Work out the finished part from the listing and answer in its coordinate system (mm). A direction names the side the tool comes from. Coordinates: 2 decimals unless noted, no trailing zeros. Loops run counter-clockwise (first coordinate to the right, second up) from the corner with the lowest first, then second, coordinate; pieces in that order, holes last. Notation, with made-up numbers: (60, 0) - (119, 0) arc R22 cw to (119, 39) - close; hole circle Ø6 at (-17.5, -0.5). An arc over 180 degrees is marked (long way). Write each question's results on one line, items separated by ' | '. Start each with the question number.
1. A cutting plane is placed at A-A on y = 2. Determine the outline of the cut face in (x, z), then the cut area to 3 significant figures.
2. Find the intervals of material crossed by line 1 along X through (y, z) = (16.25, 14); line 2 along Z through (x, y) = (-13, 6.25); line 3 along X through (y, z) = (16, 14), in increasing order. Write a range as [from, to].
3. A cutting plane is placed at B-B on x = -5.5. Determine the outline of the cut face in (y, z).
4. A cutting plane is placed at C-C on x = -23.5. Determine the outline of the cut face in (y, z), then the cut area to 3 significant figures.
5. A cutting plane is placed at D-D on y = 12.75. Determine the outline of the cut face in (x, z), then the cut area to 3 significant figures.
6. Each of these flat-tipped pins is pushed along its axis until it touches: P1, Ø6.5, axis at y = 12.5, z = 6.5, coming from the +X side; P2, Ø3, axis at y = 13.5, z = 22.5, coming from the +X side; P3, Ø3, axis at x = 3.5, y = 11.5, coming from the +Z side. Where does it stop, or does it pass through?
7. Determine the mould class of faces 5 (the flat face through (0, 8, 7)), 6 (the cylindrical face through (-53.986, 8.451, 5.703)), 7 (the flat face through (-8, 9, 11)), 8 (the flat face through (-20, 8, 0)) for opening direction X: released by +X, released by -X, zero draft, split by the parting line, or undercut.
8. Which of the six approach directions +Z, -Z, +X, -X, +Y, -Y give full straight-line access (tool end or side, diameter ignored) to faces 1 (the flat face through (-11.5, 9, 13)), 2 (the flat face through (-46.054, 8.619, 14.368)), 3 (the flat face through (-56, 8, 25)), 4 (the flat face through (-25, 8, 15))?
from build123d import *

# Parameters (mm, degrees)
SALIENTE_EXTRUIR1_DEPTH  = 17
CORTAR_EXTRUIR3_DEPTH    = 40
CORTAR_REVOLUCI_N1_ANGLE = 90
CORTAR_EXTRUIR4_DEPTH    = 10
CORTAR_EXTRUIR5_DEPTH    = 27
CROQUIS15_W              = 6
CROQUIS15_H              = 17
SALIENTE_EXTRUIR2_DEPTH  = 7
CROQUIS16_W              = 2
CROQUIS16_H              = 17
SALIENTE_EXTRUIR3_DEPTH  = 7
CORTAR_EXTRUIR6_START    = -23
CROQUIS17_W              = 8
CROQUIS17_H              = 4
CORTAR_EXTRUIR6_DEPTH    = 23


with BuildPart() as part:
    # Croquis1 → Saliente-Extruir1 (new body)
    with BuildSketch(Plane(origin=(0, 0, 0), x_dir=(1, 0, 0), z_dir=(0, 1, 0))):
        with BuildLine():
            Line((0, 0), (-40, 0))
            ThreePointArc((-40, 0), (-54.142135624, -5.857864376), (-60, -20))
            Line((-60, -20), (-60, -25))
            Line((-60, -25), (0, -25))
            Line((0, -25), (0, 0))
        make_face()
    extrude(amount=SALIENTE_EXTRUIR1_DEPTH)

    # Croquis8 → Cortar-Extruir3 (cut)
    with BuildSketch(Plane(origin=(0, 0, 0), x_dir=(0, 0, -1), z_dir=(1, 0, 0))):
        with BuildLine():
            Line((-5, 0), (0, 0))
            Line((0, 0), (0, 5))
            ThreePointArc((0, 5), (-1.464466094, 1.464466094), (-5, 0))
        make_face()
        with BuildLine():
            Line((0, 12), (0, 17))
            Line((0, 17), (-5, 17))
            ThreePointArc((-5, 17), (-1.464466094, 15.535533906), (0, 12))
        make_face()
    extrude(amount=-CORTAR_EXTRUIR3_DEPTH, mode=Mode.SUBTRACT)

    # Croquis13 → Cortar-Revolución1 (revolve, cut)
    with BuildSketch(Plane(origin=(-40, 0, 0), x_dir=(0, 0, -1), z_dir=(1, 0, 0))):
        with BuildLine():
            Line((-5, 17), (0, 17))
            Line((0, 17), (0, 12))
            ThreePointArc((0, 12), (-1.464466094, 15.535533906), (-5, 17))
        make_face()
        with BuildLine():
            Line((0, 5), (0, 0))
            Line((0, 0), (-5, 0))
            ThreePointArc((-5, 0), (-1.464466094, 1.464466094), (0, 5))
        make_face()
    revolve(axis=Axis((-40, 22.120784126, 20), (0, 1, 0)), revolution_arc=CORTAR_REVOLUCI_N1_ANGLE, mode=Mode.SUBTRACT)

    # Croquis14 → Cortar-Extruir4 (cut)
    with BuildSketch(Plane(origin=(0, 0, 20), x_dir=(-1, 0, 0), z_dir=(0, 0, -1))):
        with BuildLine():
            Line((55, 17), (60, 17))
            Line((60, 17), (60, 12))
            ThreePointArc((60, 12), (58.535533906, 15.535533906), (55, 17))
        make_face()
        with BuildLine():
            Line((60, 5), (60, 0))
            Line((60, 0), (55, 0))
            ThreePointArc((55, 0), (58.535533906, 1.464466094), (60, 5))
        make_face()
    extrude(amount=-CORTAR_EXTRUIR4_DEPTH, mode=Mode.SUBTRACT)

    # Croquis12 → Cortar-Extruir5 (cut)
    with BuildSketch(Plane(origin=(0, 17, 0), x_dir=(1, 0, 0), z_dir=(0, 1, 0))):
        with BuildLine():
            Line((0, -15), (-39, -15))
            ThreePointArc((-39, -15), (-43.242640687, -16.757359313), (-45, -21))
            Line((-45, -21), (-45, -25))
            Line((-45, -25), (0, -25))
            Line((0, -25), (0, -15))
        make_face()
    extrude(amount=-CORTAR_EXTRUIR5_DEPTH, mode=Mode.SUBTRACT)

    # Croquis15 → Saliente-Extruir2 (add)
    with BuildSketch(Plane.XY.offset(25)):
        with Locations((-48, 8.5)):
            Rectangle(CROQUIS15_W, CROQUIS15_H)
    extrude(amount=SALIENTE_EXTRUIR2_DEPTH)

    # Croquis16 → Saliente-Extruir3 (add)
    with BuildSketch(Plane(origin=(0, 0, 0), x_dir=(0, 0, -1), z_dir=(1, 0, 0))):
        with Locations((-14, 8.5)):
            Rectangle(CROQUIS16_W, CROQUIS16_H)
    extrude(amount=SALIENTE_EXTRUIR3_DEPTH)

    # Croquis17 → Cortar-Extruir6 (cut)
    with BuildSketch(Plane.XZ.offset(CORTAR_EXTRUIR6_START)):
        with Locations((-7.5, 13)):
            Rectangle(CROQUIS17_W, CROQUIS17_H)
        with BuildLine():
            Line((-45, 21), (-48.843271123, 17.156728877))
            Line((-48.843271123, 17.156728877), (-43.186416873, 11.499874628))
            Line((-43.186416873, 11.499874628), (-39.650882968, 15.035408533))
            ThreePointArc((-39.650882968, 15.035408533), (-43.466838804, 16.994085486), (-45, 21))
        make_face()
    extrude(amount=CORTAR_EXTRUIR6_DEPTH, mode=Mode.SUBTRACT)


solid = part.part
Values:
1) outline: (-59, 20) arc R19 ccw to (-40, 1) - (0, 1) - (0, 13) - (7, 13) - (7, 15) - (-3.5, 15) - (-3.5, 11) - (-11.5, 11) - (-11.5, 15) - (-39, 15) arc R6 cw to (-39.65, 15.04) - (-43.19, 11.5) - (-48.84, 17.16) - (-45, 21) - (-45, 32) - (-51, 32) - (-51, 25) - (-59, 25) - close | area: 887 mm^2
2) line 1: [-56.58, -45.69], [-40.69, -11.5], [-3.5, 7] | line 2: [0, 15] | line 3: [-56.97, -45.69], [-40.69, -11.5], [-3.5, 7]
3) outline: (0, 5) arc R5 ccw to (5, 0) - (12, 0) arc R5 ccw to (17, 5) - (17, 11) - (0, 11) - close
4) outline: (0, 5) arc R5 ccw to (5, 0) - (12, 0) arc R5 ccw to (17, 5) - (17, 15) - (0, 15) - close | area: 244 mm^2
5) outline: (-59.94, 20) arc R19.94 ccw to (-40, 0.06) - (0, 0.06) - (0, 13) - (7, 13) - (7, 15) - (-3.5, 15) - (-3.5, 11) - (-11.5, 11) - (-11.5, 15) - (-39, 15) arc R6 cw to (-39.65, 15.04) - (-43.19, 11.5) - (-48.84, 17.16) - (-45, 21) - (-45, 32) - (-51, 32) - (-51, 25) - (-59.94, 25) - close | area: 958 mm^2
6) P1: x = 0 | P2: x = -45 | P3: z = 15
7) face 5: released by +X | face 6: released by -X | face 7: undercut | face 8: zero draft
8) face 1: +Z, +Y, -Y | face 2: +Y, -Y | face 3: +Z, -X, +Y, -Y | face 4: +Z, +X, +Y, -Y
